Can you work these out from the model? Positions are in its coordinate system, mm. A direction names the side the tool comes from. Coordinates: 2 decimals unless noted, no trailing zeros. Write each loop counter-clockwise with the first axis right and the second up, starting at its lowest first coordinate (ties: lowest second). Pieces come first, ordered by that corner, then holes. Notation, with made-up numbers: (2.25, -34) - (14.25, -34) arc R22 cw to (14.25, -4) - close; hole circle Ø10 at (-1.75, 74.25). An arc over 180 degrees is marked (long way). Write each question's results on one line, items separated by ' | '. Start each with the question number.
```python
from build123d import *


with BuildPart() as part:
    # Szkic2 → Obrót1 (revolve)
    with BuildSketch(Plane.XY, mode=Mode.PRIVATE) as obr_t1_sk:
        Polygon((0, 10.2), (-35.5, 10.2), (-35.5, 15.9), (-30.5, 15.9), (-30.5, 58), (-28, 58), (-28, 85.767658064), (-21, 105), (0, 105), align=None)
    obr_t1 = revolve(obr_t1_sk.sketch.rotate(Axis((0, 0, 0), (-1, 0, 0)), 90), axis=Axis((0, 0, 0), (-1, 0, 0)))

    # Lustro2: Obrót1 across Right Plane
    add(obr_t1.mirror(Plane(origin=(0, 0, 0), x_dir=(0, 0, -1), z_dir=(1, 0, 0))))


solid = part.part
```
Q1. If we section it at C-C (x = 7): Please give me the cut outline in (y, z), then the cut area to 3 significant figures.
Q2. I'm going to push flat-ended pins straight in: pin 1 Ø18.5 at (y, z) = (0, 0) entering from -X; pin 2 Ø6 at (x, y) = (6.5, 83.5) entering from -Z; pin 3 Ø1.5 at (x, y) = (-1, 47) entering from -Z; pin 4 Ø1.5 at (x, z) = (15.5, 74) entering from +Y. Where does each tip first touch, or does it pass through?
Q3. If we section it at A-A (z = 0): Please give me the cut outline in (x, y).
Q4. I need wall thicknesses on line 1 along Z through (x, y) = (-15, -1); line 2 along X through (y, z) = (-51.5, 29); line 3 along X through (y, z) = (-28.5, 24.5). Which ranges of each line are inside material? Lowest first, please. Write a range as from..to.
Q5. Thinking about a two-plate mould opening in Z: for faces 4 (the face through (-32.965, -0.699, 15.885)), 5 (the face through (-30.5, 12, 12)), which applies, pulls with the +Z half, pulls with the -Z half, needs draft (parallel to the pull), parting line crosses it, or undercut?
Q6. If we section it at D-D (x = -23.5): Please give me the cut outline in (y, z).
Q7. For faces 1 (the face through (-35.5, -0.2, 10.4)), 2 (the face through (32.965, -0.699, 15.885)), 3 (the face through (-28, 56, 18)), which set-ups out of +Z, -Z, +X, -X, +Y, -Y let a thin tool reach every point of the face, with its end or its side?
Answer list:
1) outline: circle Ø210 at (0, 0); hole circle Ø20.4 at (0, 0) | area: 34,300 mm2
2) pin 1: passes through | pin 2: stops at z = -67.41 | pin 3: stops at z = -94.27 | pin 4: stops at y = 75.23
3) outline: (-35.5, -15.9) - (-30.5, -15.9) - (-30.5, -58) - (-28, -58) - (-28, -85.77) - (-21, -105) - (21, -105) - (28, -85.77) - (28, -58) - (30.5, -58) - (30.5, -15.9) - (35.5, -15.9) - (35.5, -10.2) - (-35.5, -10.2) - close; (-35.5, 10.2) - (35.5, 10.2) - (35.5, 15.9) - (30.5, 15.9) - (30.5, 58) - (28, 58) - (28, 85.77) - (21, 105) - (-21, 105) - (-28, 85.77) - (-28, 58) - (-30.5, 58) - (-30.5, 15.9) - (-35.5, 15.9) - close
4) line 1: z = -105..-10.15, 10.15..105 | line 2: x = -28..28 | line 3: x = -30.5..30.5
5) face 4: parting line crosses it | face 5: needs draft
6) outline: circle Ø196.26 at (0, 0); hole circle Ø20.4 at (0, 0)
7) face 1: +Z, -Z, -X, +Y, -Y | face 2: +X | face 3: -X
